```python
from build123d import *

# Parameters (mm, degrees)
EXTRUDE_1_DEPTH     = 2.6
SKETCH_2_R          = 0.65
CUT_EXTRUDE_1_DEPTH = 43.411489878
SKETCH_3_R          = 0.6
CUT_EXTRUDE_2_DEPTH = 43.675729829
SKETCH_5_W          = 0.4
SKETCH_5_H          = 0.3
CUT_EXTRUDE_3_DEPTH = 0.3
SKETCH_7_W          = 0.4
SKETCH_7_H          = 0.3
CUT_EXTRUDE_4_DEPTH = 0.3
FILLET_1_R          = 1


with BuildPart() as part:
    # 草圖1 → 填料-伸長1 (new body)
    with BuildSketch(Plane.XY):
        Polygon((6.798471119, 23.329620726), (6.798471119, 26.429618372), (-2.663246867, 26.429618372), (-2.663246867, 38.429618372), (6.810322616, 38.429618372), (6.810322616, 41.529620726), (-8.189677384, 41.529620726), (-8.201528881, 23.329620726), align=None)
    extrude(amount=EXTRUDE_1_DEPTH)

    # 草圖2 → 除料-伸長1 (cut, through all)
    with BuildSketch(Plane.XY.offset(2.6)):
        with Locations((-7.000552109, 24.829620726)):
            Circle(SKETCH_2_R)
        with Locations((-7.000552109, 27.329620726)):
            Circle(SKETCH_2_R)
        with Locations((-7.000552109, 40.029620726)):
            Circle(SKETCH_2_R)
        with Locations((-7.000552109, 37.529620726)):
            Circle(SKETCH_2_R)
    extrude(amount=-CUT_EXTRUDE_1_DEPTH, mode=Mode.SUBTRACT)

    # 草圖3 → 除料-伸長2 (cut, through all)
    with BuildSketch(Plane(origin=(-2.663246867, 0, 0), x_dir=(0, 0, -1), z_dir=(1, 0, 0))):
        with Locations(Location((-1.65, 34.929620726, 0), (0, 0, 90))):
            Circle(SKETCH_3_R)
        with Locations(Location((-1.65, 29.929620726, 0), (0, 0, 90))):
            Circle(SKETCH_3_R)
    extrude(amount=-CUT_EXTRUDE_2_DEPTH, mode=Mode.SUBTRACT)

    # 草圖5 → 除料-伸長3 (cut)
    with BuildSketch(Plane(origin=(-8.216717207, 0.005350572, 0), x_dir=(0, 0, 1), z_dir=(-0.9999997879816068, 0.0006511810359147792, 0))):
        with Locations((2.4, 34.924278959)):
            Rectangle(SKETCH_5_W, SKETCH_5_H)
        with Locations((2.4, 29.924278959)):
            Rectangle(SKETCH_5_W, SKETCH_5_H)
    extrude(amount=-CUT_EXTRUDE_3_DEPTH, mode=Mode.SUBTRACT)

    # 草圖7 → 除料-伸長4 (cut)
    with BuildSketch(Plane(origin=(-2.663246867, 0, 0), x_dir=(0, 0, -1), z_dir=(1, 0, 0))):
        with Locations((-2.4, 29.929620726)):
            Rectangle(SKETCH_7_W, SKETCH_7_H)
        with Locations((-2.4, 34.929620726)):
            Rectangle(SKETCH_7_W, SKETCH_7_H)
    extrude(amount=-CUT_EXTRUDE_4_DEPTH, mode=Mode.SUBTRACT)

    # 圓角1
    fillet_1_edges = [part.edges().sort_by_distance(p)[0] for p in [
        (-2.663246867, 38.429618372, 1.3),
        (-2.663246867, 26.429618372, 1.3),
    ]]
    fillet(fillet_1_edges, radius=FILLET_1_R)


solid = part.part
```
CAD build for the part. Positions are in the model's coordinates, mm. A direction names the side the tool comes from. Give positions to 0.01 mm unless a question says otherwise; leave off trailing zeros. Loops run counter-clockwise (first coordinate to the right, second up) from the corner with the lowest first, then second, coordinate; pieces in that order, holes last. Notation, with made-up numbers: M 83,5.25 L 100,5.25 A8 cw 100,16.25 Z; hole C -1,49 d8. An arc over 180 degrees is marked long. Use one line per item in the form item = value.
Item 1: Slice it at B-B (x = 2.5). List the corners of the cut face in (y, z).
Determined:
outline = M 23.33,0 L 26.43,0 L 26.43,2.6 L 23.33,2.6 Z; M 38.43,0 L 41.53,0 L 41.53,2.6 L 38.43,2.6 Z
Item 2: Flat gauge pins, fed straight in: pin 1 (1 mm diameter, centred on y = 29.5, z = 1, fed in from -X); pin 2 (0.8 mm diameter, centred on y = 24.5, z = 1, fed in from +X). Where does each tip first touch, or does it go through?
Determined:
pin_1 = -8.2
pin_2 = 6.8
Item 3: Slice it at C-C (x = -4.75). List the corners of the cut face in (y, z), plus the area to 3 significant figures.
Determined:
outline = M 23.33,0 L 41.53,0 L 41.53,2.6 L 23.33,2.6 Z; hole C 29.93,1.65 d1.2; hole C 34.93,1.65 d1.2
area = 45.1 mm2
Item 4: Two-plate mould, pull along X, no slides. Class faces 1 (the face through (-2.663, 32, 1)), 2 (the face through (-7.085, 27.974, 1.318)), 3 (the face through (3, 38.43, 1)): pulls with the +X half, pulls with the -X half, needs draft (parallel to the pull), parting line crosses it, or undercut.
Determined:
face_1 = pulls with the +X half
face_2 = undercut
face_3 = needs draft
Item 5: Which spindle directions (+Z, -Z, +X, -X, +Y, -Y) get a long thin tool onto all of the face, cutting with end or side? Do faces 4 (the face through (3, 26.43, 1)), 5 (the face through (6.81, 40, 1)). Say none if no direction does.
Determined:
face_4 = +Z, -Z, +X
face_5 = +Z, -Z, +X, +Y, -Y
Item 6: Slice it at A-A (z = 1.65). List the corners of the cut face in (x, y).
Determined:
outline = M -8.2,23.33 L 6.8,23.33 L 6.8,26.43 L -1.66,26.43 A1 cw -2.66,27.43 L -2.66,29.33 L -8.2,29.33 Z; M -8.2,30.53 L -2.66,30.53 L -2.66,34.33 L -8.19,34.33 Z; M -8.19,35.53 L -2.66,35.53 L -2.66,37.43 A1 cw -1.66,38.43 L 6.81,38.43 L 6.81,41.53 L -8.19,41.53 Z; hole C -7,24.83 d1.3; hole C -7,27.33 d1.3; hole C -7,37.53 d1.3; hole C -7,40.03 d1.3
Item 7: Drill centre lines: probe 1 along Y at (x, z) = (0.25, 1.1); probe 2 along Y at (x, z) = (-4.75, 1.65); probe 3 along Y at (x, z) = (-6, 1.35). Where is each one in solid material? Low to high. Write a range as from..to.
Determined:
probe_1 = 23.33..26.43, 38.43..41.53
probe_2 = 23.33..29.33, 30.53..34.33, 35.53..41.53
probe_3 = 23.33..29.41, 30.45..34.41, 35.45..41.53
Item 8: Slice it at D-D (y = 24.5). List the corners of the cut face in (x, z).
Determined:
outline = M -8.2,0 L -7.56,0 L -7.56,2.6 L -8.2,2.6 Z; M -6.44,0 L 6.8,0 L 6.8,2.6 L -6.44,2.6 Z
